Geometry check sheet. Reference: the model listing, model coordinates, mm. Coordinates: 2 decimals unless noted, no trailing zeros. Order: outer loops, then holes, each group sorted by start corner. A loop starts at its lowest first (then second) coordinate and runs counter-clockwise, first axis right, second up. Notation, with made-up numbers: (73, 67.25) -> (108, 67.25) arc R15 cw to (108, 90.25) -> close; hole circle Ø5 at (65, 58.5). An arc over 180 degrees is marked (long way). Answer as CSV lines item,"result". Start each with the question number.
from build123d import *

# Parameters (mm, degrees)
CYLINDER110_R          = 1.6
CYLINDER110_DEPTH      = 10
CYLINDER111_R          = 1.6
CYLINDER111_DEPTH      = 10
BOX050_W               = 20
BOX050_H               = 6
BOX050_DEPTH           = 20
CUT058_PLACEMENT_ANGLE = 90


with BuildPart() as cylinder110:
    # Cylinder110 → Cylinder110 (new body)
    with BuildSketch(Plane(origin=(320, 26, 0), x_dir=(1, 0, 0), z_dir=(0, -1, 0))):
        Circle(CYLINDER110_R)
    extrude(amount=CYLINDER110_DEPTH)


with BuildPart() as fusion097:
    # Cylinder111 → Cylinder111 (new body)
    with BuildSketch(Plane(origin=(320, 26, 10), x_dir=(1, 0, 0), z_dir=(0, -1, 0))):
        Circle(CYLINDER111_R)
    extrude(amount=CYLINDER111_DEPTH)

    # Fusion097: union Cylinder110
    add(cylinder110.part)


with BuildPart() as fusion097_1:
    # Fusion097 placement: moved
    add(fusion097.part.moved(Location((15, -1.5, 6))))


with BuildPart() as cut058:
    # Box050 → Box050 (new body)
    with BuildSketch(Plane(origin=(320, 18.5, 1.5), x_dir=(1, 0, 0), z_dir=(0, 0, 1))):
        with Locations((10, 3)):
            Rectangle(BOX050_W, BOX050_H)
    extrude(amount=BOX050_DEPTH)

    # Cut058: cut Fusion097
    add(fusion097_1.part, mode=Mode.SUBTRACT)


with BuildPart() as cut058_1:
    # Cut058 placement: moved
    add(cut058.part.moved(Location((320, 37.5, 343))).rotate(Axis((320, 37.5, 343), (0, 1, 0)), CUT058_PLACEMENT_ANGLE))


solid = cut058_1.part
Q1. Release check for a two-part mould opening along Z. For faces 1 (the flat face through (331, 62, 13)), 2 (the cylindrical face through (327.586, 59.042, 8.208)), 3 (the flat face through (331, 59, 23)) record: released by +Z, released by -Z, zero draft, split by the parting line, or undercut.
Q2. Sectioned sample at A-A, the plane x = 336. Record the cut outline in (y, z), then the cut area to 3 significant figures.
Q3. Sectioned sample at C-C, the plane y = 60.45. Record the cut outline in (x, z), then the cut area to 3 significant figures.
Q4. Sectioned sample at B-B, the plane z = 8. Record the cut outline in (x, y).
Q5. Thickness scan on L1, parallel to X at y = 57.7, z = 8; L2, parallel to X at y = 61.65, z = 8.75; L3, parallel to Z at x = 325, y = 60.05. Record the ranges inside material, lowest first.
Geometry results:
1,face 1,"zero draft"
1,face 2,"undercut"
1,face 3,"released by +Z"
2,outline,"(56, 3) -> (62, 3) -> (62, 6.4) -> (56, 6.4) -> close; (56, 9.6) -> (62, 9.6) -> (62, 23) -> (56, 23) -> close"
2,area,"101 mm^2"
3,outline,"(321.5, 3) -> (341.5, 3) -> (341.5, 23) -> (321.5, 23) -> close; hole circle Ø3.2 at (326, 8); hole circle Ø3.2 at (336, 8)"
3,area,"384 mm^2"
4,outline,"(321.5, 56) -> (324.4, 56) -> (324.4, 62) -> (321.5, 62) -> close; (327.6, 56) -> (334.4, 56) -> (334.4, 62) -> (327.6, 62) -> close; (337.6, 56) -> (341.5, 56) -> (341.5, 62) -> (337.6, 62) -> close"
5,L1,"x = 321.5 to 324.4, 327.6 to 334.4, 337.6 to 341.5"
5,L2,"x = 321.5 to 324.59, 327.41 to 334.59, 337.41 to 341.5"
5,L3,"z = 3 to 6.75, 9.25 to 23"
